```python
from build123d import *

# Parameters (mm, degrees)
SKIZZE1_W                       = 46
SKIZZE1_H                       = 28
AUFSATZ_LINEAR_AUSTRAGEN1_DEPTH = 7
SKIZZE2_R                       = 8.075
SCHNITT_LINEAR_AUSTRAGEN1_DEPTH = 5.6
AUFSATZ_LINEAR_START            = 0.5
SKIZZE10_R                      = 8.075
SKIZZE10_R_2                    = 6.625
AUFSATZ_LINEAR_AUSTRAGEN2_DEPTH = 0.5
VERRUNDUNG1_R                   = 2
SKIZZE11_R                      = 2.2
SCHNITT_LINEAR_AUSTRAGEN8_DEPTH = 8
FASE1_SIZE                      = 0.5


with BuildPart() as part:
    # Skizze1 → Aufsatz-Linear austragen1 (new body)
    with BuildSketch(Plane.XY):
        Rectangle(SKIZZE1_W, SKIZZE1_H)
    extrude(amount=AUFSATZ_LINEAR_AUSTRAGEN1_DEPTH)

    # Skizze2 → Schnitt-Linear austragen1 (cut)
    with BuildSketch(Plane.XY.offset(7)):
        with Locations((0, 4.65)):
            Circle(SKIZZE2_R)
    extrude(amount=-SCHNITT_LINEAR_AUSTRAGEN1_DEPTH, mode=Mode.SUBTRACT)

    # Skizze10 → Aufsatz-Linear austragen2 (add)
    with BuildSketch(Plane.XY.offset(1.4).offset(AUFSATZ_LINEAR_START)):
        with Locations((0, 4.65)):
            Circle(SKIZZE10_R)
        with Locations((0, 4.65)):
            Circle(SKIZZE10_R_2, mode=Mode.SUBTRACT)
    extrude(amount=-AUFSATZ_LINEAR_AUSTRAGEN2_DEPTH)

    # Verrundung1
    verrundung1_edges = [part.edges().sort_by_distance(p)[0] for p in [
        (23, -14, 3.5),
        (-23, -14, 3.5),
        (-23, 14, 3.5),
        (23, 14, 3.5),
    ]]
    fillet(verrundung1_edges, radius=VERRUNDUNG1_R)

    # Skizze11 → Schnitt-Linear austragen8 (cut)
    with BuildSketch(Plane.XZ.offset(14)):
        with Locations(Location((0, 3.5, 0), (0, 0, 270))):
            Circle(SKIZZE11_R)
    extrude(amount=-SCHNITT_LINEAR_AUSTRAGEN8_DEPTH, mode=Mode.SUBTRACT)

    # Fase1
    fase1_edges = [part.edges().sort_by_distance(p)[0] for p in [
        (-8.075, 4.65, 7),
        (0, 14, 0),
        (0, 14, 7),
        (23, 0, 0),
        (0, -14, 0),
        (-23, 0, 0),
        (-22.414213562, -13.414213562, 0),
        (-22.414213562, 13.414213562, 0),
        (22.414213562, -13.414213562, 0),
        (22.414213562, 13.414213562, 0),
        (23, 0, 7),
        (-23, 0, 7),
        (0, -14, 7),
        (-22.414213562, -13.414213562, 7),
        (-22.414213562, 13.414213562, 7),
        (22.414213562, -13.414213562, 7),
        (22.414213562, 13.414213562, 7),
    ]]
    chamfer(fase1_edges, length=FASE1_SIZE)


solid = part.part
```
Here's how the part is built. I have some questions about the finished solid (model axes, mm). A direction names the side the tool comes from. Coordinates: 2 decimals unless noted, no trailing zeros. Write each loop counter-clockwise with the first axis right and the second up, starting at its lowest first coordinate (ties: lowest second). Pieces come first, ordered by that corner, then holes. Notation, with made-up numbers: M -1,3 L 26,3 A26 cw 26,36 Z; hole C 89.5,6.5 d8. An arc over 180 degrees is marked long. Answer as CSV lines item,"result". Start each with the question number.
Q1. If we mould it in two halves opening along X, with no side actions, what happens to faces 1 (the cylindrical face through (-22.43, -13.4, 3.54)), 2 (the flat face through (0, -6, 4)), 3 (the flat face through (0, -14, 1))? For each: pulls with the +X half, pulls with the -X half, needs draft (parallel to the pull), parting line crosses it, or undercut.
Q2. Will these pins go through, and if not, where does the flat tip stop? pin 1 Ø5 at (x, y) = (2, 7.5) entering from +Z; pin 2 Ø1 at (x, y) = (5, 9) entering from +Z; pin 3 Ø2 at (x, z) = (1, 4) entering from -Y.
Q3. Suppose I cut it at A-A, the plane y = -6.5. List the corners of the cut face in (x, z) for me.
Q4. Suppose I cut it at C-C, the plane x = 0. List the corners of the cut face in (y, z) for me (3 decimals), then the cut area to 3 significant figures.
Q5. Suppose I cut it at B-B, the plane z = 2.5. List the corners of the cut face in (x, y) for me (3 decimals), then the cut area to 3 significant figures.
Q6. Suppose I cut it at D-D, the plane y = 4.65. List the corners of the cut face in (x, z) for me (3 decimals).
Q7. I need wall thicknesses on probe 1 along Y at (x, z) = (0, 1.6) (3 decimals); probe 2 along Y at (x, z) = (-6, 5.5); probe 3 along X at (y, z) = (-12.5, 3.5). Which ranges of each line are inside material? Lowest first, please. Write a range as [from, to].
Q8. For faces 4 (the cylindrical face through (0.66, -10.06, 1.4)), 5 (the conical face through (-22.144, -13.169, 0.135)), 6 (the flat face through (0, 5, 1.4)), which set-ups out of +Z, -Z, +X, -X, +Y, -Y let a thin tool reach every point of the face, with its end or its side?
Entries:
1,face 1,"pulls with the -X half"
1,face 2,"undercut"
1,face 3,"needs draft"
2,pin 1,"stops at z = 1.4"
2,pin 2,"stops at z = 1.9"
2,pin 3,"stops at y = -6"
3,outline,"M -23,0.5 L -22.5,0 L 22.5,0 L 23,0.5 L 23,6.5 L 22.5,7 L -22.5,7 L -23,6.5 Z; hole C 0,3.5 d4.4"
4,outline,"M -14,0.5 L -13.5,0 L 13.5,0 L 14,0.5 L 14,6.5 L 13.5,7 L 13.225,7 L 12.725,6.5 L 12.725,1.9 L 11.275,1.9 L 11.275,1.4 L -1.975,1.4 L -1.975,1.9 L -3.425,1.9 L -3.425,6.5 L -3.925,7 L -13.5,7 L -14,6.5 L -14,5.7 L -6,5.7 L -6,1.3 L -14,1.3 Z"
4,area,"71.1 mm²"
5,outline,"M -23,-12 A2 ccw -21,-14 L -1.96,-14 L -1.96,-6 L 1.96,-6 L 1.96,-14 L 21,-14 A2 ccw 23,-12 L 23,12 A2 ccw 21,14 L -21,14 A2 ccw -23,12 Z; hole C 0,4.65 d16.15"
5,area,"1,050 mm²"
6,outline,"M -23,0.5 L -22.5,0 L 22.5,0 L 23,0.5 L 23,6.5 L 22.5,7 L 8.575,7 L 8.075,6.5 L 8.075,1.9 L 6.625,1.9 L 6.625,1.4 L -6.625,1.4 L -6.625,1.9 L -8.075,1.9 L -8.075,6.5 L -8.575,7 L -22.5,7 L -23,6.5 Z"
7,probe 1,"y = [-6, -1.975], [11.275, 14]"
7,probe 2,"y = [-14, -0.75], [10.05, 14]"
7,probe 3,"x = [-22.94, -2.2], [2.2, 22.94]"
8,face 4,"-Y"
8,face 5,"-Z, -X, -Y"
8,face 6,"+Z"
